from build123d import *

# Parameters (mm, degrees)
BOSS_EXTRUDE1_DEPTH = 5
BOSS_EXTRUDE2_DEPTH = 15
SKETCH3_W           = 5
SKETCH3_H           = 35
BOSS_EXTRUDE3_DEPTH = 15
SKETCH4_W           = 5
SKETCH4_H           = 35
BOSS_EXTRUDE4_DEPTH = 5
BOSS_EXTRUDE5_DEPTH = 5
SKETCH7_R           = 1.8
CUT_EXTRUDE1_DEPTH  = 6
SKETCH9_W           = 5
SKETCH9_H           = 15
BOSS_EXTRUDE6_DEPTH = 13
BOSS_EXTRUDE7_DEPTH = 4
SKETCH13_R          = 1.5
CUT_EXTRUDE4_DEPTH  = 40


with BuildPart() as part:
    # Sketch1 → Boss-Extrude1 (new body)
    with BuildSketch(Plane.XY):
        Polygon((-7.529880478, -25.806772908), (27.470119522, -25.806772908), (27.470119522, -10.806772908), (7.470119522, -10.806772908), (7.470119522, 9.193227092), (-7.529880478, 9.193227092), align=None)
    extrude(amount=BOSS_EXTRUDE1_DEPTH)



with BuildPart() as body_2:
    # Sketch2 → Boss-Extrude2 (new body)
    with BuildSketch(Plane(origin=(0, 0, 0), x_dir=(-1, 0, 0), z_dir=(0, 0, -1))):
        Polygon((-7.470119522, 9.193227092), (-12.470119522, 9.193227092), (-12.470119522, -5.806772908), (-27.470119522, -5.806772908), (-27.470119522, -10.806772908), (-7.470119522, -10.806772908), align=None)
    extrude(amount=BOSS_EXTRUDE2_DEPTH)


with BuildPart() as body_3:
    # Sketch3 → Boss-Extrude3 (new body)
    with BuildSketch(Plane(origin=(0, 0, 0), x_dir=(-1, 0, 0), z_dir=(0, 0, -1))):
        with Locations((10.029880478, -8.306772908)):
            Rectangle(SKETCH3_W, SKETCH3_H)
    extrude(amount=BOSS_EXTRUDE3_DEPTH)


with BuildPart() as part_1:
    add(part.part)

    add(body_3.part)  # Boss-Extrude4 merges body 3
    # Sketch4 → Boss-Extrude4 (add)
    with BuildSketch(Plane.XY):
        with Locations((-10.029880478, -8.306772908)):
            Rectangle(SKETCH4_W, SKETCH4_H)
    extrude(amount=BOSS_EXTRUDE4_DEPTH)


    add(body_2.part)  # Boss-Extrude5 merges body 2
    # Sketch5 → Boss-Extrude5 (add)
    with BuildSketch(Plane.XY):
        Polygon((7.470119522, 9.193227092), (7.470119522, -10.806772908), (27.470119522, -10.806772908), (27.470119522, -5.806772908), (12.470119522, -5.806772908), (12.470119522, 9.193227092), align=None)
    extrude(amount=BOSS_EXTRUDE5_DEPTH)

    # Sketch7 → Cut-Extrude1 (cut, through all)
    with BuildSketch(Plane(origin=(0, 0, 0), x_dir=(-1, 0, 0), z_dir=(0, 0, -1))):
        with Locations((0.029880478, 1.693227092)):
            Circle(SKETCH7_R)
        with Locations((-17.470119522, -18.306772908)):
            Circle(SKETCH7_R)
    extrude(amount=-CUT_EXTRUDE1_DEPTH, mode=Mode.SUBTRACT)

    # Sketch9 → Boss-Extrude6 (add)
    with BuildSketch(Plane(origin=(0, 0, -15), x_dir=(-1, 0, 0), z_dir=(0, 0, -1))):
        with Locations((10.029880478, -18.306772908)):
            Rectangle(SKETCH9_W, SKETCH9_H)
    extrude(amount=BOSS_EXTRUDE6_DEPTH)

    # Sketch12 → Boss-Extrude7 (add)
    with BuildSketch(Plane.XZ.offset(25.806772908)):
        Polygon((7.470119522, -28), (-12.529880478, -28), (-12.529880478, 5), (7.470119522, 5), (27.470119522, 5), (27.470119522, -15), (7.470119522, -15), align=None)
    extrude(amount=BOSS_EXTRUDE7_DEPTH)

    # Sketch13 → Cut-Extrude4 (cut, through all)
    with BuildSketch(Plane.XZ.offset(29.806772908)):
        with Locations((-0.029880478, -20.5)):
            Circle(SKETCH13_R)
    extrude(amount=-CUT_EXTRUDE4_DEPTH, mode=Mode.SUBTRACT)


solid = part_1.part
Could you check a few things on this model? Use its own coordinates, in mm. A direction names the side the tool comes from. Give positions to 0.01 mm unless a question says otherwise; leave off trailing zeros. Order: outer loops, then holes, each group sorted by start corner. A loop starts at its lowest first (then second) coordinate and runs counter-clockwise, first axis right, second up.
1. Suppose I cut it at A-A (z = -20.5). List the corners of the cut face in (x, y) for me, plus the area to 3 significant figures.
2. For faces 4 (the flat face through (20, -5.807, -5)), 5 (the flat face through (-10, -10.807, -21)), 6 (the flat face through (18, -10.807, -7)), 7 (the flat face through (-7.53, -12, -11)), 8 (the flat face through (7.47, -28, -21)), which set-ups out of +Z, -Z, +X, -X, +Y, -Y let a thin tool reach every point of the face, with its end or its side?
3. Suppose I cut it at B-B (y = -4). List the corners of the cut face in (x, z) for me.
4. Suppose I cut it at C-C (x = 15). List the corners of the cut face in (y, z) for me, plus the area to 3 significant figures.
5. I need wall thicknesses on L1, parallel to X at y = 4.5, z = -7; L2, parallel to Y at x = 16, z = -1; L3, parallel to X at y = -22, z = -5. Which ranges of each line are inside material? Lowest first, please.
6. We'd pull the mould along Y, two halves only. Please class faces 1 (the flat face through (12.47, 2, -5)), 2 (the cylindrical face through (16.64, -19.904, 2.465)), 3 (the flat face through (0, 9.193, 2)): pulls with the +Y half, pulls with the -Y half, needs draft (parallel to the pull), parting line crosses it, or undercut.
7. Will these pins go through, and if not, where does the flat tip stop? P1, Ø1, axis at x = -5, z = -19.5, coming from the +Y side; P2, Ø4, axis at x = 12, y = -9.5, coming from the -Z side; P3, Ø4, axis at x = 1, y = 3, coming from the -Z side.
8. Suppose I cut it at D-D (z = -6.5). List the corners of the cut face in (x, y) for me, plus the area to 3 significant figures.
Solved:
1. outline: (-12.53, -29.81) - (-1.53, -29.81) - (-1.53, -25.81) - (-7.53, -25.81) - (-7.53, -10.81) - (-12.53, -10.81) - close; (1.47, -29.81) - (7.47, -29.81) - (7.47, -25.81) - (1.47, -25.81) - close
1. area: 143 mm2
2. face 4: +Z, -Z, +X, +Y
2. face 5: -Z, +X, -X, +Y
2. face 6: -Z, +X
2. face 7: -Z, +Y
2. face 8: -Z, +X, +Y, -Y
3. outline: (-12.53, -15) - (-7.53, -15) - (-7.53, 0) - (7.47, 0) - (7.47, -15) - (12.47, -15) - (12.47, 5) - (-12.53, 5) - close
4. outline: (-29.81, -15) - (-25.81, -15) - (-25.81, 0) - (-10.81, 0) - (-10.81, -15) - (-5.81, -15) - (-5.81, 5) - (-29.81, 5) - close
4. area: 255 mm2
5. L1: x = -12.53 to -7.53, 7.47 to 12.47
5. L2: y = -29.81 to -25.81, -10.81 to -5.81
5. L3: x = -12.53 to -7.53
6. face 1: needs draft
6. face 2: undercut
6. face 3: pulls with the +Y half
7. P1: stops at y = -25.81
7. P2: stops at z = -15
7. P3: stops at z = 0
8. outline: (-12.53, -29.81) - (27.47, -29.81) - (27.47, -25.81) - (-7.53, -25.81) - (-7.53, 9.19) - (-12.53, 9.19) - close; (7.47, -10.81) - (27.47, -10.81) - (27.47, -5.81) - (12.47, -5.81) - (12.47, 9.19) - (7.47, 9.19) - close
8. area: 510 mm2
